For this review, take the finished solid that the model builds, in its own axes (mm). Round coordinates to 2 decimals unless told otherwise and drop trailing zeros. One line per item, written item: value. Start each with the question number.
Q1. Add section A-A on z = 5. Give the number of separate pieces and of enclosed holes in the cut face, and give its area (3 significant figures).
Q2. Clearance check with flat-ended pins moving along their axes: pin 1 Ø3 at (x, z) = (556.5, 4) entering from -Y; pin 2 Ø3 at (x, z) = (333, 5) entering from +Y (3 decimals). State where each tip first meets the part, or that it passes through.
Q3. For probe 1 along Y at (x, z) = (558.8, 1.5) (1 decimal); probe 2 along Y at (x, z) = (318.5, 0.75) (3 decimals); probe 3 along Y at (x, z) = (137, 2.5) (3 decimals), list the stretches that pass through material, from the lowest coordinate up.
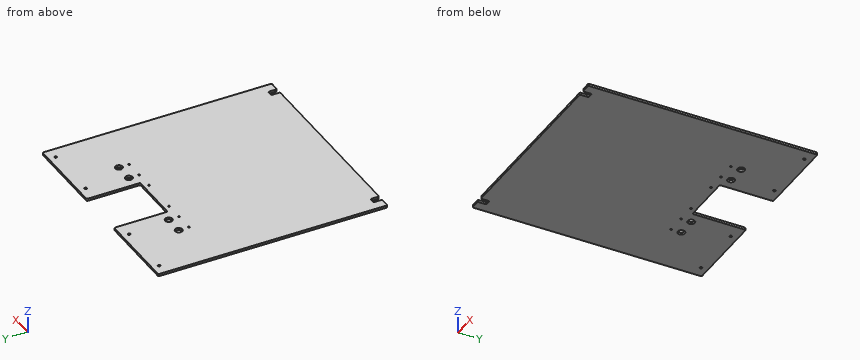
```python
from build123d import *

# Parameters (mm, degrees)
SKETCH1_W                        = 590.55
SKETCH1_H                        = 479.425
BOSS_EXTRUDE1_DEPTH              = 6.35
SKETCH2_W                        = 15.875
SKETCH2_H                        = 23.8125
CUT_EXTRUDE1_DEPTH               = 761.682559038
F_10_0_1935_DIAMETER_HOLE1_D     = 4.9149
SKETCH6_W                        = 225.425
SKETCH6_H                        = 146.05
BOSS_EXTRUDE3_DEPTH              = 6.35
F_49_64_0_76563_DIAMETER_HOLE1_D = 19.447002
F_1_4_CLEARANCE_HOLE1_D          = 6.7564
FILLET1_R                        = 3.302


with BuildPart() as part:
    # Sketch1 → Boss-Extrude1 (new body)
    with BuildSketch(Plane.XY):
        with Locations((295.275, 239.7125)):
            Rectangle(SKETCH1_W, SKETCH1_H)
    extrude(amount=BOSS_EXTRUDE1_DEPTH)

    # Sketch2 → Cut-Extrude1 (cut, through all)
    with BuildSketch(Plane.XY.offset(6.35)):
        with Locations((34.925, 11.90625)):
            Rectangle(SKETCH2_W, SKETCH2_H)
        with Locations((555.625, 11.90625)):
            Rectangle(SKETCH2_W, SKETCH2_H)
    extrude(amount=-CUT_EXTRUDE1_DEPTH, mode=Mode.SUBTRACT)

    # #10 (0.1935) Diameter Hole1 (through all)
    with Locations(Plane.XY.offset(6.35)):
        with Locations((142.875, 465.507832), (244.475, 465.507832), (346.075, 465.507832), (447.675, 465.507832), (193.675, 465.507832), (396.875, 465.507832)):
            Hole(F_10_0_1935_DIAMETER_HOLE1_D / 2)

    # Sketch6 → Boss-Extrude3 (add)
    with BuildSketch(Plane.XY.offset(6.35)):
        with Locations((477.8375, 552.45)):
            Rectangle(SKETCH6_W, SKETCH6_H)
        with Locations((112.7125, 552.45)):
            Rectangle(SKETCH6_W, SKETCH6_H)
    extrude(amount=-BOSS_EXTRUDE3_DEPTH)

    # 49/64 (0.76563) Diameter Hole1 (through all)
    with Locations(Plane.XY.offset(6.35)):
        with Locations((142.875, 493.342168), (447.675, 493.342168), (193.675, 493.342168), (396.875, 493.342168)):
            Hole(F_49_64_0_76563_DIAMETER_HOLE1_D / 2)

    # 1/4 Clearance Hole1 (through all)
    with Locations(Plane.XY.offset(6.35)):
        with Locations((31.75, 606.425), (184.15, 606.425), (406.4, 606.425), (558.8, 606.425)):
            Hole(F_1_4_CLEARANCE_HOLE1_D / 2)

    # Fillet1
    fillet1_edges = [part.edges().sort_by_distance(p)[0] for p in [
        (42.8625, 0, 3.175),
        (26.9875, 0, 3.175),
        (26.9875, 23.8125, 3.175),
        (42.8625, 23.8125, 3.175),
        (563.5625, 0, 3.175),
        (547.6875, 0, 3.175),
        (547.6875, 23.8125, 3.175),
        (563.5625, 23.8125, 3.175),
        (590.55, 0, 3.175),
        (365.125, 625.475, 3.175),
        (365.125, 479.425, 3.175),
        (590.55, 625.475, 3.175),
        (0, 0, 3.175),
        (225.425, 479.425, 3.175),
        (225.425, 625.475, 3.175),
        (0, 625.475, 3.175),
    ]]
    fillet(fillet1_edges, radius=FILLET1_R)


solid = part.part
```
Result set:
1. separate pieces: 1
1. enclosed holes: 14
1. area: 347,000 mm^2
2. pin 1: stops at y = 23.81
2. pin 2: stops at y = 479.425
3. probe 1: y = 23.8 to 603, 609.8 to 625.5
3. probe 2: y = 0 to 479.425
3. probe 3: y = 0 to 485.594, 501.09 to 625.475
